Verification items for the finished model (mm, model axes). Give positions to 0.01 mm unless a question says otherwise; leave off trailing zeros. Write each loop counter-clockwise with the first axis right and the second up, starting at its lowest first coordinate (ties: lowest second). Pieces come first, ordered by that corner, then holes.
Autodesk Inventor part; units mm, degrees
ref_plane "YZ Plane" through (0, 0, 0) normal (1, 0, 0) x (0, 1, 0)
ref_plane "XZ Plane" through (0, 0, 0) normal (0, 1, 0) x (-1, 0, 0)
ref_plane "XY Plane" through (0, 0, 0) normal (0, 0, 1) x (1, 0, 0)
sketch "Sketch1" plane through (0, 0, 0) normal (0, 0, 1) x (1, 0, 0)
  line L0 (-4.0005, 1.27) -> (4.0005, 1.27)
  line L1 (4.0005, 1.27) -> (4.0005, -1.27)
  line L2 (4.0005, -1.27) -> (-4.0005, -1.27)
  line L3 (-4.0005, -1.27) -> (-4.0005, 1.27)
  line L4 (0, 0) -> (-4.0005, 0) construction
  line L5 (0, 0) -> (0, -1.27) construction
  line L6 (0, 0) -> (0, 1.27) construction
  line L7 (0, 0) -> (4.0005, 0) construction
  dimension "d0" = 8.001
  dimension "d1" = 2.54
extrude "Extrusion1" add sketch "Sketch1" along normal blind 8.509
sketch "Sketch2" plane through (0, 0, 8.509) normal (0, 0, 1) x (1, 0, 0)
  line L0 (-4.0005, 1.27) -> (4.0005, 1.27)
  line L1 (-4.0005, -1.27) -> (-4.0005, 1.27)
  line L2 (-2.794, 0.3175) -> (-2.159, 0.3175)
  line L3 (-2.159, 0.3175) -> (-2.159, -0.3175)
  line L4 (-2.159, -0.3175) -> (-2.794, -0.3175)
  line L5 (-2.794, -0.3175) -> (-2.794, 0.3175)
  dimension "d4" = 0.635
  dimension "d5" = 1.2065
  dimension "d6" = 0.9525
extrude "Extrusion2" cut sketch "Sketch2" against normal blind 6.35
chamfer "Chamfer1" distance 0.381 angle 45 4 edges at (-2.4765, 0.3175, 8.509) (-2.159, 0, 8.509) (-2.4765, -0.3175, 8.509) (-2.794, 0, 8.509)
sketch "Sketch3" plane through (0, 0, 2.159) normal (0, 0, 1) x (1, 0, 0)
  line L0 (-2.794, 0.3175) -> (-2.794, -0.3175)
  line L1 (-2.794, -0.3175) -> (-2.794, 0.3175)
  line L2 (-2.794, 0.3175) -> (-2.159, 0.3175)
  line L3 (-2.159, 0.3175) -> (-2.159, -0.3175)
  line L4 (-2.159, -0.3175) -> (-2.794, -0.3175)
extrude "Extrusion3" add sketch "Sketch3" against normal blind 5.08
pattern_linear "Rectangular Pattern3" count 3 spacing 2.54 along (1, 0, 0) of "Extrusion2", "Chamfer1"
pattern_linear "Rectangular Pattern4" count 3 spacing 2.54 along (1, 0, 0) of "Extrusion3"
properties part number "1x3 Header Connector" material "ABS Plastic"
Item 1: Sectioned sample at B-B on z = 7.25. Record the cut outline in (x, y).
Answer key:
outline: (-4, -1.27) - (4, -1.27) - (4, 1.27) - (-4, 1.27) - close; hole (-2.79, -0.32) - (-2.16, -0.32) - (-2.16, 0.32) - (-2.79, 0.32) - close; hole (-0.25, -0.32) - (0.38, -0.32) - (0.38, 0.32) - (-0.25, 0.32) - close; hole (2.29, -0.32) - (2.92, -0.32) - (2.92, 0.32) - (2.29, 0.32) - close
Item 2: Scan lines: line 1 along X through (y, z) = (-0.05, 2.75); line 2 along Y through (x, z) = (2.5, 2.25); line 3 along Z through (x, y) = (1.25, 0.25). Record each from-to range of solid material in increasing order.
Answer key:
line 1: x = -4 to -2.79, -2.16 to -0.25, 0.38 to 2.29, 2.92 to 4
line 2: y = -1.27 to -0.32, 0.32 to 1.27
line 3: z = 0 to 8.51
Item 3: Sectioned sample at A-A on z = -1. Record the cut outline in (x, y), then the cut area to 3 significant figures.
Answer key:
outline: (-2.79, -0.32) - (-2.16, -0.32) - (-2.16, 0.32) - (-2.79, 0.32) - close; (-0.25, -0.32) - (0.38, -0.32) - (0.38, 0.32) - (-0.25, 0.32) - close; (2.29, -0.32) - (2.92, -0.32) - (2.92, 0.32) - (2.29, 0.32) - close
area: 1.21 mm2
Item 4: Sectioned sample at D-D on x = -3. Record the cut outline in (y, z), then the cut area to 3 significant figures.
Answer key:
outline: (-1.27, 0) - (1.27, 0) - (1.27, 8.51) - (0.7, 8.51) - (0.52, 8.33) - (-0.52, 8.33) - (-0.7, 8.51) - (-1.27, 8.51) - close
area: 21.4 mm2
Item 5: Depth check by flat-ended pin: pin 1 (0.8 mm diameter, centred on x = 0.5, y = 0, fed in from -Z); pin 2 (0.5 mm diameter, centred on y = 0, z = -1.5, fed in from +X); pin 3 (0.5 mm diameter, centred on x = 2.5, y = 0, fed in from +Z). Enter the tip coordinate at first touch or a pass-through.
Answer key:
pin 1: stops at z = -2.92
pin 2: stops at x = 2.92
pin 3: stops at z = 8.16
